from build123d import *

# Parameters (mm, degrees)
F1_DEPTH = 25
F2_W     = 31.581489
F2_H     = 47.974935
F3_DEPTH = 6.5


with BuildPart() as f1:
    # F0 (on Front) → F1 (new body, symmetric)
    with BuildSketch(Plane.XZ):
        Polygon((0, 33), (0, 0), (63, 0), (63, 20), (31, 20), (31, 58), (25, 58), align=None)
    extrude(amount=F1_DEPTH, both=True)

    # F2 (on Front) → F3 (cut, symmetric)
    with BuildSketch(Plane.XZ):
        with Locations((53.790744, 10.887097)):
            Rectangle(F2_W, F2_H)
    extrude(amount=F3_DEPTH, both=True, mode=Mode.SUBTRACT)

    # F4: F1 across plane


with BuildPart() as f1_1:
    add(f1.part)
    add(f1.part.mirror(Plane.YZ))


solid = f1_1.part
Verification items for the finished model (mm, model axes). A direction names the side the tool comes from. Give positions to 0.01 mm unless a question says otherwise; leave off trailing zeros. Order: outer loops, then holes, each group sorted by start corner. A loop starts at its lowest first (then second) coordinate and runs counter-clockwise, first axis right, second up. Notation, with made-up numbers: M 33.25,52.5 L 66.25,52.5 A29 ccw 66.25,72.5 Z; hole C 6,57.25 d1. An arc over 180 degrees is marked long. Answer as a JSON object with one key per item and string values. Group by question number.
1) Access from +Z, -Z, +X, -X, +Y, -Y to the whole of each face (thin tool, end or side, straight path). Record for faces 5 (the face through (50, 6.5, 10)), 6 (the face through (37, 0, 20)), 7 (the face through (13, 0, 46)), 8 (the face through (-37, 0, 20)).
2) Depth check by flat-ended pin: pin 1 Ø6 at (y, z) = (20, 23.5) entering from -X; pin 2 Ø10.5 at (y, z) = (0, 5.5) entering from +X; pin 3 Ø8 at (x, y) = (20.5, -13.5) entering from +Z. Enter the tip coordinate at first touch or a pass-through.
3) Cross-section at C-C (y = 11.5). Enter the section's corners in (x, z), then the cut area to 3 significant figures.
4) Cross-section at B-B (x = 40). Enter the section's corners in (y, z).
5) Cross-section at D-D (z = 5). Enter the section's corners in (x, y), then the cut area to 3 significant figures.
6) Mould release check, pull along Y, two halves, no side actions. Record for faces 1 (the face through (1, 25, 23)), 2 (the face through (-50, -6.5, 10)), 3 (the face through (63, 16, 10)), 4 (the face through (-50, 6.5, 10)): released by +Y, released by -Y, zero draft, split by the parting line, or undercut.
7) Cross-section at A-A (z = 53). Enter the section's corners in (x, y).
8) Scan lines: line 1 along X through (y, z) = (15, 39.5); line 2 along Y through (x, z) = (52, 11.5); line 3 along Z through (x, y) = (-48.5, -10). Record each from-to range of solid material in increasing order. Write a range as [from, to].
Result sheet:
{
 "1": {"face 5": "+Z, -Z, +X", "face 6": "+Z, +X, +Y, -Y", "face 7": "+Z, +Y, -Y", "face 8": "+Z, -X, +Y, -Y"},
 "2": {"pin 1": "stops at x = -31", "pin 2": "stops at x = 38", "pin 3": "stops at z = 57.5"},
 "3": {"outline": "M -63,0 L 63,0 L 63,20 L 31,20 L 31,58 L 25,58 L 0,33 L -25,58 L -31,58 L -31,20 L -63,20 Z", "area": "4,250 mm2"},
 "4": {"outline": "M -25,0 L -6.5,0 L -6.5,20 L -25,20 Z; M 6.5,0 L 25,0 L 25,20 L 6.5,20 Z"},
 "5": {"outline": "M -63,-25 L 63,-25 L 63,-6.5 L 38,-6.5 L 38,6.5 L 63,6.5 L 63,25 L -63,25 L -63,6.5 L -38,6.5 L -38,-6.5 L -63,-6.5 Z", "area": "5,650 mm2"},
 "6": {"face 1": "released by +Y", "face 2": "undercut", "face 3": "zero draft", "face 4": "undercut"},
 "7": {"outline": "M -31,-25 L -20,-25 L -20,25 L -31,25 Z; M 20,-25 L 31,-25 L 31,25 L 20,25 Z"},
 "8": {"line 1": "x = [-31, -6.5], [6.5, 31]", "line 2": "y = [-25, -6.5], [6.5, 25]", "line 3": "z = [0, 20]"}
}
